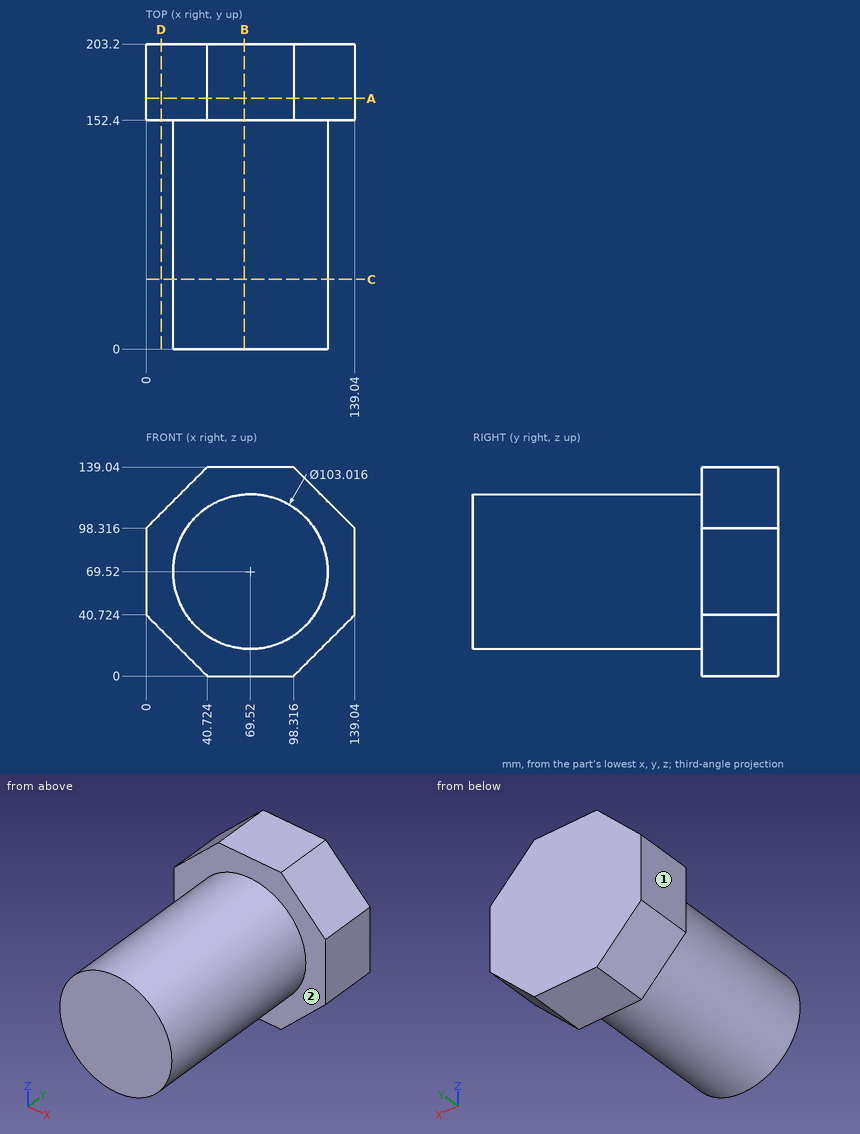
Geometry: see drawing. Coordinates: mm, zero at the bounding-box minimum. A direction names the side the tool comes from. Coordinates: 2 decimals unless noted, no trailing zeros. Write each loop counter-clockwise with the first axis right and the second up, starting at its lowest first coordinate (ties: lowest second). Pieces come first, ordered by that corner, then holes.
1) Pin query (flat end, axial travel): pin 1 Ø1 at (x, y) = (99, 161.5) entering from -Z (1 decimal); pin 2 Ø1 at (y, z) = (89, 108.5) entering from -X; pin 3 Ø1 at (x, y) = (87.5, 111.5) entering from -Z. Return the tip coordinate at first contact, or that it passes through.
2) Section D-D on x = 10. Output: boundary loops of the cut face in (y, z).
3) Section A-A on y = 167. Output: boundary loops of the cut face in (x, z), and give its area (3 significant figures).
4) Section B-B on x = 65.5. Output: boundary loops of the cut face in (y, z).
5) Set-up query: the marked faces 1 and 2. Return all of +Z, -Z, +X, -X, +Y, -Y with unobstructed straight access to the full face (end or side cutting, diameter ignored); none if empty.
6) Material intervals for line 1 along Y through (x, z) = (30, 108); line 2 along Z through (x, y) = (29, 39); line 3 along Z through (x, y) = (77, 52), sorted ascending.
7) Section C-C on y = 46.5. Output: boundary loops of the cut face in (x, z) (1 decimal), and give its area (4 significant figures).
Check result:
1. pin 1: stops at z = 0.2
1. pin 2: stops at x = 35.28
1. pin 3: stops at z = 21.07
2. outline: (152.4, 30.72) - (203.2, 30.72) - (203.2, 108.32) - (152.4, 108.32) - close
3. outline: (0, 40.72) - (40.72, 0) - (98.32, 0) - (139.04, 40.72) - (139.04, 98.32) - (98.32, 139.04) - (40.72, 139.04) - (0, 98.32) - close
3. area: 16,000 mm2
4. outline: (0, 18.17) - (152.4, 18.17) - (152.4, 0) - (203.2, 0) - (203.2, 139.04) - (152.4, 139.04) - (152.4, 120.87) - (0, 120.87) - close
5. face 1: +Z, -Z, -X, +Y, -Y
5. face 2: -Y
6. line 1: y = 152.4 to 203.2
6. line 2: z = 37.72 to 101.32
6. line 3: z = 18.56 to 120.48
7. outline: circle Ø103 at (69.5, 69.5)
7. area: 8,335 mm2
